```python
from build123d import *

# Parameters (mm, degrees)
BOX008_W          = 0.5
BOX008_H          = 3.25
BOX008_DEPTH      = 3.5
BOX010_W          = 0.5
BOX010_H          = 3.25
BOX010_DEPTH      = 3.5
BOX009_W          = 0.5
BOX009_H          = 3.25
BOX009_DEPTH      = 3.5
CYLINDER009_R     = 1.25
CYLINDER009_DEPTH = 6.5
CYLINDER008_R     = 1.25
CYLINDER008_DEPTH = 6.5
BOX007_W          = 20
BOX007_H          = 6.5
BOX007_DEPTH      = 11


with BuildPart() as obj1:
    # Box008 → Box008 (new body)
    with BuildSketch(Plane(origin=(4.75, 1.625, -6.5), x_dir=(1, 0, 0), z_dir=(0, 0, 1))):
        with Locations((0.25, 1.625)):
            Rectangle(BOX008_W, BOX008_H)
    extrude(amount=BOX008_DEPTH)


with BuildPart() as obj2:
    # Box010 → Box010 (new body)
    with BuildSketch(Plane(origin=(-3.25, 1.625, -6.5), x_dir=(1, 0, 0), z_dir=(0, 0, 1))):
        with Locations((0.25, 1.625)):
            Rectangle(BOX010_W, BOX010_H)
    extrude(amount=BOX010_DEPTH)


with BuildPart() as obj3:
    # Box009 → Box009 (new body)
    with BuildSketch(Plane(origin=(12.75, 1.625, -6.5), x_dir=(1, 0, 0), z_dir=(0, 0, 1))):
        with Locations((0.25, 1.625)):
            Rectangle(BOX009_W, BOX009_H)
    extrude(amount=BOX009_DEPTH)


with BuildPart() as limitswitchmountinghole002:
    # Cylinder009 → Cylinder009 (new body)
    with BuildSketch(Plane(origin=(9.5, 0, 0), x_dir=(1, 0, 0), z_dir=(0, 1, 0))):
        Circle(CYLINDER009_R)
    extrude(amount=CYLINDER009_DEPTH)


with BuildPart() as limitswitchmountinghole001:
    # Cylinder008 → Cylinder008 (new body)
    with BuildSketch(Plane(origin=(0, 0, 0), x_dir=(1, 0, 0), z_dir=(0, 1, 0))):
        Circle(CYLINDER008_R)
    extrude(amount=CYLINDER008_DEPTH)


with BuildPart() as obj4:
    # Box007 → Box007 (new body)
    with BuildSketch(Plane(origin=(-5.25, 0, -3), x_dir=(1, 0, 0), z_dir=(0, 0, 1))):
        with Locations((10, 3.25)):
            Rectangle(BOX007_W, BOX007_H)
    extrude(amount=BOX007_DEPTH)

    # Cut007: cut LimitSwitchMountingHole001
    add(limitswitchmountinghole001.part, mode=Mode.SUBTRACT)

    # Cut008: cut LimitSwitchMountingHole002
    add(limitswitchmountinghole002.part, mode=Mode.SUBTRACT)

    # Fusion005: union obj1, obj2, obj3
    add(obj1.part)
    add(obj2.part)
    add(obj3.part)


solid = obj4.part
```
Build history of the part. All positions in model axes, mm. A direction names the side the tool comes from. Round coordinates to 2 decimals unless told otherwise and drop trailing zeros. Loops run counter-clockwise (first coordinate to the right, second up) from the corner with the lowest first, then second, coordinate; pieces in that order, holes last.
Item 1: Pin check, flat tips, straight feed: P1, Ø2.5, axis at y = 3.5, z = -4, coming from the +X side; P2, Ø2.5, axis at y = 3.5, z = -4.5, coming from the +X side; P3, Ø2.5, axis at y = 3, z = -5.5, coming from the -X side; P4, Ø1.5, axis at x = 9.5, z = 0, coming from the +Y side. Stop position of each tip, or through.
Item 2: Which spindle directions (+Z, -Z, +X, -X, +Y, -Y) get a long thin tool onto all of the face, cutting with end or side? Do faces 1 (the face through (-2.75, 3, -5)), 2 (the face through (-3.25, 3, -5)), 3 (the face through (8.25, 3.2, -0.05)). Say none if no direction does.
Item 3: Saw through at A-A (y = 3.25). List the corners of the cut face in (x, z), then the cut area to 3 significant figures.
Item 4: Drill centre lines: line 1 along X through (y, z) = (2.75, -4.5); line 2 along X through (y, z) = (4.5, 0); line 3 along Z through (x, y) = (0, 3.5). Where is each one in solid material? Low to high.
Item 5: Saw through at B-B (z = 0). List the corners of the cut face in (x, y), then the cut area to 3 significant figures.
Item 6: Two-plate mould, pull along X, no slides. Class faces 4 (the face through (13.25, 3, -5)), 5 (the face through (5.25, 3, -5)), 6 (the face through (5, 6.5, 2)): released by +X, released by -X, zero draft, split by the parting line, or undercut.
Item 7: Saw through at D-D (z = -3.75). List the corners of the cut face in (x, y) (3 decimals).
Item 8: Saw through at C-C (x = 0). List the corners of the cut face in (y, z).
Worked answers:
1. P1: stops at x = 14.75
1. P2: stops at x = 13.25
1. P3: stops at x = -3.25
1. P4: passes through
2. face 1: -Z, +Y, -Y
2. face 2: -Z, -X, +Y, -Y
2. face 3: +Y, -Y
3. outline: (-5.25, -3) - (-3.25, -3) - (-3.25, -6.5) - (-2.75, -6.5) - (-2.75, -3) - (4.75, -3) - (4.75, -6.5) - (5.25, -6.5) - (5.25, -3) - (12.75, -3) - (12.75, -6.5) - (13.25, -6.5) - (13.25, -3) - (14.75, -3) - (14.75, 8) - (-5.25, 8) - close; hole circle Ø2.5 at (0, 0); hole circle Ø2.5 at (9.5, 0)
3. area: 215 mm2
4. line 1: x = -3.25 to -2.75, 4.75 to 5.25, 12.75 to 13.25
4. line 2: x = -5.25 to -1.25, 1.25 to 8.25, 10.75 to 14.75
4. line 3: z = -3 to -1.25, 1.25 to 8
5. outline: (-5.25, 0) - (-1.25, 0) - (-1.25, 6.5) - (-5.25, 6.5) - close; (1.25, 0) - (8.25, 0) - (8.25, 6.5) - (1.25, 6.5) - close; (10.75, 0) - (14.75, 0) - (14.75, 6.5) - (10.75, 6.5) - close
5. area: 97.5 mm2
6. face 4: released by +X
6. face 5: undercut
6. face 6: zero draft
7. outline: (-3.25, 1.625) - (-2.75, 1.625) - (-2.75, 4.875) - (-3.25, 4.875) - close; (4.75, 1.625) - (5.25, 1.625) - (5.25, 4.875) - (4.75, 4.875) - close; (12.75, 1.625) - (13.25, 1.625) - (13.25, 4.875) - (12.75, 4.875) - close
8. outline: (0, -3) - (6.5, -3) - (6.5, -1.25) - (0, -1.25) - close; (0, 1.25) - (6.5, 1.25) - (6.5, 8) - (0, 8) - close
